```python
from build123d import *
from OCP.BRepFilletAPI import BRepFilletAPI_MakeChamfer

# Parameters (mm, degrees)
SKIZZE1_W                           = 37.5
SKIZZE1_H                           = 20
AUFSATZ_LINEAR_AUSTRAGEN1_DEPTH     = 40.8
SKIZZE2_W                           = 2.5
SKIZZE2_H                           = 19
AUFSATZ_LINEAR_AUSTRAGEN2_DEPTH     = 6.8
F_4_3_4_3_DIAMETER_HOLE2_AT_2_COUNT = 2
F_4_3_4_3_DIAMETER_HOLE2_AT_2_PITCH = 10
CUT_EXTRUDE1_REACH                  = 58.886
SKETCH1_W                           = 3
SKETCH1_H                           = 2.5
BOSS_EXTRUDE1_DEPTH                 = 0.55
SKIZZE5_R                           = 6.5
AUFSATZ_LINEAR_AUSTRAGEN3_DEPTH     = 1.3
SKIZZE6_R                           = 3
AUFSATZ_LINEAR_AUSTRAGEN4_DEPTH     = 4
SKIZZE7_W                           = 4
SKIZZE7_H                           = 6
AUFSATZ_LINEAR_AUSTRAGEN5_DEPTH     = 1.5
SKIZZE8_W                           = 2.7
SKIZZE8_H                           = 5
SKIZZE8_W_2                         = 1.7
SKIZZE8_H_2                         = 4
AUFSATZ_LINEAR_AUSTRAGEN6_DEPTH     = 5
F_5_0_5_DIAMETER_HOLE1_D            = 5
F_5_0_5_DIAMETER_HOLE1_DEPTH        = 3.5
F_5_0_5_DIAMETER_HOLE1_TIP          = 1.502151548
M3_GEWINDEBOHRUNG1_D                = 2.5
M3_GEWINDEBOHRUNG1_DEPTH            = 8.5
M3_GEWINDEBOHRUNG1_TIP              = 0.751075774
CHAMFER1_SIZE                       = 1.5
CHAMFER1_SIZE_2                     = 2.5


with BuildPart() as part:
    # Skizze1 → Aufsatz-Linear austragen1 (new body)
    with BuildSketch(Plane.XY):
        Rectangle(SKIZZE1_W, SKIZZE1_H)
    extrude(amount=AUFSATZ_LINEAR_AUSTRAGEN1_DEPTH)

    # Skizze2 → Aufsatz-Linear austragen2 (add)
    with BuildSketch(Plane.XY.offset(40.8)):
        with Locations((9.5, 0)):
            Rectangle(SKIZZE2_W, SKIZZE2_H)
    aufsatz_linear_austragen2 = extrude(amount=AUFSATZ_LINEAR_AUSTRAGEN2_DEPTH)

    # Skizze3 → Ø4.3 (4.3) Diameter Hole2 (revolve, cut)
    with BuildSketch(Plane(origin=(10.75, 5, 44.2), x_dir=(0, 0, -1), z_dir=(0, 1, 0))):
        Polygon((0, 0), (0, 11.291850331), (2.15, 10), (2.15, 0), align=None)
    f_4_3_4_3_diameter_hole2 = revolve(axis=Axis((17.1, 5, 44.2), (-1, 0, 0)), mode=Mode.SUBTRACT)

    # Ø4.3 (4.3) Diameter Hole2 at 2: Ø4.3 (4.3) Diameter Hole2 ×2
    with Locations(*[(0, -i * F_4_3_4_3_DIAMETER_HOLE2_AT_2_PITCH, 0) for i in range(1, F_4_3_4_3_DIAMETER_HOLE2_AT_2_COUNT)]):
        add(f_4_3_4_3_diameter_hole2, mode=Mode.SUBTRACT)

    # Sketch1 → Cut-Extrude1 (cut, up to next)
    with BuildSketch(Plane(origin=(10.75, 0, 0), x_dir=(0, 0, -1), z_dir=(1, 0, 0)), mode=Mode.PRIVATE) as cut_extrude1_sk1:
        with Locations((-47.05, 5)):
            Rectangle(SKETCH1_W, SKETCH1_H)
    cut_extrude1_tool1 = extrude(cut_extrude1_sk1.sketch, amount=-CUT_EXTRUDE1_REACH, mode=Mode.PRIVATE) & part.part
    # Sketch1 → Cut-Extrude1 (cut, up to next)
    with BuildSketch(Plane(origin=(10.75, 0, 0), x_dir=(0, 0, -1), z_dir=(1, 0, 0)), mode=Mode.PRIVATE) as cut_extrude1_sk2:
        with Locations((-47.05, -5)):
            Rectangle(SKETCH1_W, SKETCH1_H)
    cut_extrude1_tool2 = extrude(cut_extrude1_sk2.sketch, amount=-CUT_EXTRUDE1_REACH, mode=Mode.PRIVATE) & part.part
    cut_extrude1_1 = cut_extrude1_tool1.solids().sort_by_distance((10.75, 5, 47.05))[0]
    add(cut_extrude1_1, mode=Mode.SUBTRACT)
    cut_extrude1_2 = cut_extrude1_tool2.solids().sort_by_distance((10.75, -5, 47.05))[0]
    add(cut_extrude1_2, mode=Mode.SUBTRACT)
    cut_extrude1 = cut_extrude1_1 + cut_extrude1_2  # Cut-Extrude1 as one shape, for the pattern or mirror that repeats it

    # Spiegeln2: Aufsatz-Linear austragen2, Ø4.3 (4.3) Diameter Hole2, Cut-Extrude1 across plane
    add(aufsatz_linear_austragen2.mirror(Plane(origin=(0, 0, 20.4), x_dir=(1, 0, 0), z_dir=(0, 0, -1))))
    add(f_4_3_4_3_diameter_hole2.mirror(Plane(origin=(0, 0, 20.4), x_dir=(1, 0, 0), z_dir=(0, 0, -1))), mode=Mode.SUBTRACT)
    add(cut_extrude1.mirror(Plane(origin=(0, 0, 20.4), x_dir=(1, 0, 0), z_dir=(0, 0, -1))), mode=Mode.SUBTRACT)

    # Spiegeln2 copy 1 sketch → Spiegeln2 copy 1 (revolve, cut)
    with BuildSketch(Plane(origin=(10.75, -5, -3.4), x_dir=(0, 0, 1), z_dir=(0, 1, 0))):
        Polygon((0, 0), (0, -11.291850331), (2.15, -10), (2.15, 0), align=None)
    revolve(axis=Axis((17.1, -5, -3.4), (1, 0, 0)), mode=Mode.SUBTRACT)

    # Sketch3 → Boss-Extrude1 (add, symmetric)
    with BuildSketch(Plane(origin=(0, 0, 0), x_dir=(1, 0, 0), z_dir=(0, 1, 0))):
        Polygon((10.75, 0), (11.85, 0), (10.75, 6.8), align=None)
    boss_extrude1 = extrude(amount=BOSS_EXTRUDE1_DEPTH, both=True)

    # Skizze5 → Aufsatz-Linear austragen3 (add)
    with BuildSketch(Plane(origin=(18.75, 0, 0), x_dir=(0, 0, -1), z_dir=(1, 0, 0))):
        with Locations(Location((-10, 0, 0), (0, 0, 270))):
            Circle(SKIZZE5_R)
    extrude(amount=AUFSATZ_LINEAR_AUSTRAGEN3_DEPTH)

    # Skizze6 → Aufsatz-Linear austragen4 (add)
    with BuildSketch(Plane(origin=(20.05, 0, 0), x_dir=(0, 0, -1), z_dir=(1, 0, 0))):
        with Locations(Location((-10, 0, 0), (0, 0, 90))):
            Circle(SKIZZE6_R)
    extrude(amount=AUFSATZ_LINEAR_AUSTRAGEN4_DEPTH)

    # Skizze7 → Aufsatz-Linear austragen5 (add)
    with BuildSketch(Plane(origin=(0, 0, 0), x_dir=(-1, 0, 0), z_dir=(0, 0, -1))):
        with Locations((14.25, 0)):
            Rectangle(SKIZZE7_W, SKIZZE7_H)
    extrude(amount=AUFSATZ_LINEAR_AUSTRAGEN5_DEPTH)

    # Skizze8 → Aufsatz-Linear austragen6 (add)
    with BuildSketch(Plane(origin=(0, 0, -1.5), x_dir=(-1, 0, 0), z_dir=(0, 0, -1))):
        with Locations((14.25, 0)):
            Rectangle(SKIZZE8_W, SKIZZE8_H)
        with Locations((14.25, 0)):
            Rectangle(SKIZZE8_W_2, SKIZZE8_H_2, mode=Mode.SUBTRACT)
    extrude(amount=AUFSATZ_LINEAR_AUSTRAGEN6_DEPTH)

    # Ø5.0 (5) Diameter Hole1
    with Locations(Plane(origin=(0, 0, 0), x_dir=(-1, 0, 0), z_dir=(0, 0, -1))):
        with Locations((4.25, 0)):
            Hole(F_5_0_5_DIAMETER_HOLE1_D / 2, depth=F_5_0_5_DIAMETER_HOLE1_DEPTH)
            with Locations((0, 0, -(F_5_0_5_DIAMETER_HOLE1_DEPTH + F_5_0_5_DIAMETER_HOLE1_TIP / 2))):  # 118° drill point
                Cone(0, F_5_0_5_DIAMETER_HOLE1_D / 2, F_5_0_5_DIAMETER_HOLE1_TIP, mode=Mode.SUBTRACT)

    # M3 Gewindebohrung1
    with Locations(Plane(origin=(24.05, 0, 0), x_dir=(0, 0, -1), z_dir=(1, 0, 0))):
        with Locations((-10, 0)):
            Hole(M3_GEWINDEBOHRUNG1_D / 2, depth=M3_GEWINDEBOHRUNG1_DEPTH)
            with Locations((0, 0, -(M3_GEWINDEBOHRUNG1_DEPTH + M3_GEWINDEBOHRUNG1_TIP / 2))):  # 118° drill point
                Cone(0, M3_GEWINDEBOHRUNG1_D / 2, M3_GEWINDEBOHRUNG1_TIP, mode=Mode.SUBTRACT)

    # Mirror1: Boss-Extrude1 across plane
    add(boss_extrude1.mirror(Plane(origin=(0, 0, 20.4), x_dir=(1, 0, 0), z_dir=(0, 0, -1))))

    # Chamfer1
    chamfer1_edges_1 = [part.edges().sort_by_distance(p)[0] for p in [
        (-18.75, 0, 40.8),
    ]]
    chamfer1_side_1 = [part.faces().sort_by_distance(p)[0] for p in [
        (-18.75, 0, 40.77),
    ]]
    chamfer1_edges_2 = [part.edges().sort_by_distance(p)[0] for p in [
        (-18.75, 0, 0),
    ]]
    chamfer1_side_2 = [part.faces().sort_by_distance(p)[0] for p in [
        (-18.75, 0, 0.03),
    ]]
    chamfer1_edges_3 = [part.edges().sort_by_distance(p)[0] for p in [
        (-18.75, 10, 20.4),
    ]]
    chamfer1_side_3 = [part.faces().sort_by_distance(p)[0] for p in [
        (-18.72, 10, 20.4),
    ]]
    chamfer1_edges_4 = [part.edges().sort_by_distance(p)[0] for p in [
        (-18.75, -10, 20.4),
    ]]
    chamfer1_side_4 = [part.faces().sort_by_distance(p)[0] for p in [
        (-18.75, -9.97, 20.4),
    ]]
    chamfer1 = BRepFilletAPI_MakeChamfer(part.part.solid().wrapped)
    for e in chamfer1_edges_1:
        chamfer1.Add(CHAMFER1_SIZE - 0.0001, CHAMFER1_SIZE_2 - 0.0001, e.wrapped, chamfer1_side_1[0].wrapped)
    for e in chamfer1_edges_2:
        chamfer1.Add(CHAMFER1_SIZE - 0.0001, CHAMFER1_SIZE_2 - 0.0001, e.wrapped, chamfer1_side_2[0].wrapped)
    for e in chamfer1_edges_3:
        chamfer1.Add(CHAMFER1_SIZE_2 - 0.0001, CHAMFER1_SIZE - 0.0001, e.wrapped, chamfer1_side_3[0].wrapped)
    for e in chamfer1_edges_4:
        chamfer1.Add(CHAMFER1_SIZE - 0.0001, CHAMFER1_SIZE_2 - 0.0001, e.wrapped, chamfer1_side_4[0].wrapped)
    add(Compound.cast(chamfer1.Shape()), mode=Mode.REPLACE)  # a hair under: the kernel refuses the full size


solid = part.part
```
The listing builds one solid part. Answer for the finished solid, in the listing's coordinates (mm). A direction names the side the tool comes from. Coordinates: 2 decimals unless noted, no trailing zeros. Write each loop counter-clockwise with the first axis right and the second up, starting at its lowest first coordinate (ties: lowest second). Pieces come first, ordered by that corner, then holes. Notation, with made-up numbers: (37.25, -26.5) - (70.25, -26.5) arc R14 ccw to (70.25, -16.5) - close; hole circle Ø1 at (27, -3). An arc over 180 degrees is marked (long way). Return JSON: item names as keys, results as strings. Group by question number.
1. Determine the mould class of faces 5 (the flat face through (-14, 3, -1)), 6 (the flat face through (10.75, 5, -1)), 7 (the conical face through (14.93, -0.08, 9.8)) for opening direction Y: released by +Y, released by -Y, zero draft, split by the parting line, or undercut.
2. A cutting plane is placed at A-A, the plane z = -3.4. Determine the outline of the cut face in (x, y), plus the area to 3 significant figures.
3. A cutting plane is placed at C-C, the plane y = -5. Determine the outline of the cut face in (x, z), plus the area to 3 significant figures.
4. Straight lines are drawn through the part: L1, parallel to Y at x = 9.85, z = -3.4; L2, parallel to Y at x = -4, z = 2; L3, parallel to Z at x = 10.05, y = 5. For each, find the intervals that lie inside material, in ascending order.
5. Which of the six approach directions +Z, -Z, +X, -X, +Y, -Y give full straight-line access (tool end or side, diameter ignored) to faces 1 (the cylindrical face through (22.02, 2.86, 10.9)), 2 (the flat face through (10, 6.25, -6)), 3 (the flat face through (-14, 2, -4)), 4 (the flat face through (-15.6, 0, -4))?
6. A cutting plane is placed at D-D, the plane x = 0. Determine the outline of the cut face in (y, z).
7. Given pin 1 (2 mm diameter, centred on x = 4.5, y = -1, fed in from +Z); pin 2 (7 mm diameter, centred on y = 5, z = -3.4, fed in from +X); pin 3 (0.5 mm diameter, centred on x = 9, z = -5.5, fed in from -Y), each flat-ended and moving along its own axis, determine where each tip first touches the part or whether it passes through.
8. A cutting plane is placed at B-B, the plane z = 30. Determine the outline of the cut face in (x, y), plus the area to 3 significant figures.
Ans:
{
 "1": {"face 5": "released by +Y", "face 6": "zero draft", "face 7": "undercut"},
 "2": {"outline": "(-15.6, -2.5) - (-12.9, -2.5) - (-12.9, 2.5) - (-15.6, 2.5) - close; (8.25, -9.5) - (10.75, -9.5) - (10.75, -7.15) - (8.25, -7.15) - close; (8.25, -2.85) - (10.75, -2.85) - (10.75, -0.55) - (11.3, -0.55) - (11.3, 0.55) - (10.75, 0.55) - (10.75, 2.85) - (8.25, 2.85) - close; (8.25, 7.15) - (10.75, 7.15) - (10.75, 9.5) - (8.25, 9.5) - close; hole (-15.1, -2) - (-13.4, -2) - (-13.4, 2) - (-15.1, 2) - close", "area": "33.3 mm²"},
 "3": {"outline": "(-18.75, 1.5) - (-16.25, 0) - (8.25, 0) - (8.25, -1.25) - (10.75, -1.25) - (10.75, 0) - (18.75, 0) - (18.75, 5.85) - (20.05, 5.85) - (20.05, 14.15) - (18.75, 14.15) - (18.75, 40.8) - (10.75, 40.8) - (10.75, 42.05) - (8.25, 42.05) - (8.25, 40.8) - (-16.25, 40.8) - (-18.75, 39.3) - close", "area": "1,540 mm²"},
 "4": {"L1": "-9.5 to -7.15, -2.85 to 2.85, 7.15 to 9.5", "L2": "-10 to -2.49, 2.49 to 10", "L3": "-1.25 to 42.05"},
 "5": {"face 1": "+X", "face 2": "-Z, +X, -X", "face 3": "-Z", "face 4": "-Z, -X, +Y, -Y"},
 "6": {"outline": "(-10, 0) - (10, 0) - (10, 40.8) - (-10, 40.8) - close"},
 "7": {"pin 1": "z = 40.8", "pin 2": "x = 18.75", "pin 3": "y = -9.5"},
 "8": {"outline": "(-18.75, -8.5) - (-16.25, -10) - (18.75, -10) - (18.75, 10) - (-16.25, 10) - (-18.75, 8.5) - close", "area": "746 mm²"}
}
